```python
from build123d import *

# Parameters (mm, degrees)
F1_DEPTH = 19
F3_DEPTH = 10
F4_R     = 8


with BuildPart() as f1:
    # F0 (on Right) → F1 (new body)
    with BuildSketch(Plane.YZ):
        with BuildLine():
            Line((-85, 0), (0, 0))
            Line((0, 0), (0, 80))
            Line((0, 80), (-85, 80))
            ThreePointArc((-85, 80), (-102.67767, 72.67767), (-110, 55))
            Line((-110, 55), (-110, 25))
            ThreePointArc((-110, 25), (-102.67767, 7.32233), (-85, 0))
        make_face()
    extrude(amount=F1_DEPTH)

    # F2 (on face) → F3 (cut)
    with BuildSketch(Plane(origin=(0, 0, 0), x_dir=(0, -1, 0), z_dir=(-1, 0, 0))):
        with BuildLine():
            Line((57, 80), (57, 40))
            ThreePointArc((57, 40), (70, 27), (83, 40))
            Line((83, 40), (83, 80))
            Line((83, 80), (57, 80))
        make_face()
    extrude(amount=-F3_DEPTH, mode=Mode.SUBTRACT)

    # F4
    f4_edges = [f1.edges().sort_by_distance(p)[0] for p in [
        (19, -42.5, 80),
    ]]
    fillet(f4_edges, radius=F4_R)


solid = f1.part
```
Verification items for the finished model (mm, model axes). A direction names the side the tool comes from. Give positions to 0.01 mm unless a question says otherwise; leave off trailing zeros. Order: outer loops, then holes, each group sorted by start corner. A loop starts at its lowest first (then second) coordinate and runs counter-clockwise, first axis right, second up. Notation, with made-up numbers: M -15,58.25 L 30,58.25 A20 cw 30,83.25 Z; hole C -26,-13 d9. An arc over 180 degrees is marked long. Answer in a Markdown table with one row per item. Add a question column.
Item 1: Scan lines: probe 1 along X at (y, z) = (-82, 60); probe 2 along Y at (x, z) = (8.25, 62.5); probe 3 along Y at (x, z) = (4, 32). Record each from-to range of solid material in increasing order. Write a range as from..to.
Item 2: Section check A-A, the plane x = 2.25. Enter the section's corners in (y, z), and give its area (3 significant figures).
Item 3: Gauge pin test, flat ends, axial feed: pin 1 (4 mm diameter, centred on x = 16.5, z = 69, fed in from -Y); pin 2 (5 mm diameter, centred on x = 10, y = -93.5, fed in from +Z); pin 3 (2 mm diameter, centred on x = 17, z = 39, fed in from -Y) (3 decimals). Record the tip position at first contact, or that the pin passes through.
Item 4: Tool access check on faces 4 (the flat face through (5, -57, 60)), 5 (the flat face through (5, -43, 0)). Record the directions out of +Z, -Z, +X, -X, +Y, -Y that give a thin tool (end or side, any length) a straight path to the whole face; none if there is none.
Item 5: Section check D-D, the plane y = -37.5. Enter the section's corners in (x, z), and give its area (3 significant figures).
Item 6: Mould release check, pull along Y, two halves, no side actions. Record for faces 1 (the flat face through (10, -70, 54)), 2 (the flat face through (19, -52, 40)), 3 (the cylindrical face through (5.423, -102.482, 72.871)): released by +Y, released by -Y, zero draft, split by the parting line, or undercut.
Item 7: Section check C-C, the plane z = 51. Enter the section's corners in (x, y), and give its area (3 significant figures).
Item 8: Section check B-B, the plane y = -70. Enter the section's corners in (x, z).
Filled sheet:
| question | item | result |
|---|---|---|
| 1 | probe 1 | x = 10..19 |
| 1 | probe 2 | y = -108.85..-83, -57..0 |
| 1 | probe 3 | y = -110..-80.25, -59.75..0 |
| 2 | outline | M -110,25 A25 ccw -85,0 L 0,0 L 0,80 L -57,80 L -57,40 A13 cw -83,40 L -83,80 L -85,80 A25 ccw -110,55 Z |
| 2 | area | 7,230 mm^2 |
| 3 | pin 1 | stops at y = -105.29 |
| 3 | pin 2 | stops at z = 79.27 |
| 3 | pin 3 | stops at y = -108.245 |
| 4 | face 4 | +Z, -X |
| 4 | face 5 | -Z, +X, -X, +Y, -Y |
| 5 | outline | M 0,0 L 11,0 A8 ccw 19,8 L 19,72 A8 ccw 11,80 L 0,80 Z |
| 5 | area | 1,490 mm^2 |
| 6 | face 1 | undercut |
| 6 | face 2 | zero draft |
| 6 | face 3 | released by -Y |
| 7 | outline | M 0,-110 L 11,-110 A8 ccw 19,-102 L 19,0 L 0,0 L 0,-57 L 10,-57 L 10,-83 L 0,-83 Z |
| 7 | area | 1,820 mm^2 |
| 8 | outline | M 0,0 L 11,0 A8 ccw 19,8 L 19,72 A8 ccw 11,80 L 10,80 L 10,27 L 0,27 Z |
